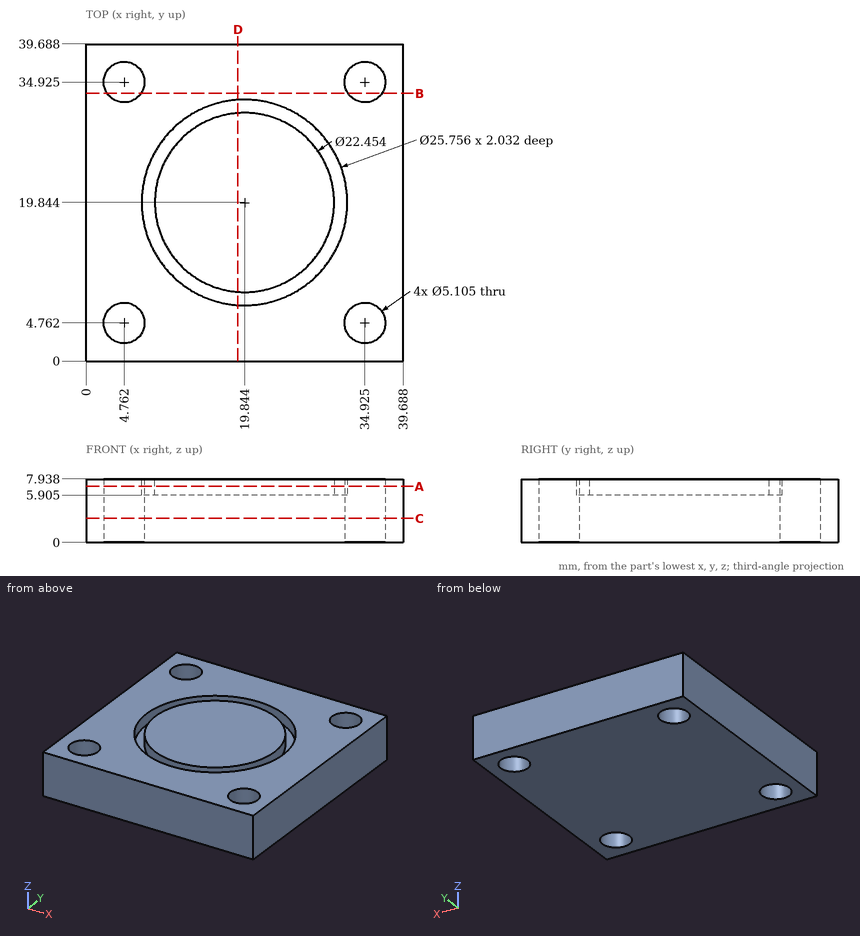
Geometry: see drawing. Coordinates: mm, zero at the bounding-box minimum. Coordinates: 2 decimals unless noted, no trailing zeros. Write each loop counter-clockwise with the first axis right and the second up, starting at its lowest first coordinate (ties: lowest second). Pieces come first, ordered by that corner, then holes. Notation, with made-up numbers: M 70,33 L 82,33 A26 ccw 82,67 Z; hole C 6.25,16.25 d7. An arc over 180 degrees is marked long. Use CSV: the item, a comma, the result in double quotes. Start each with the question number.
1. Ray query, probe 1 along X at (y, z) = (28, 7) (1 decimal); probe 2 along Y at (x, z) = (3.5, 5.5) (1 decimal); probe 3 along X at (y, z) = (34.5, 4) (1 decimal). Return the intervals inside material, ascending.
2. Cut plane C-C on z = 3. Return the cut outline in (x, y) (1 decimal), plus the area to 3 significant figures.
3. Cut plane A-A on z = 7. Return the cut outline in (x, y) (1 decimal).
4. Cut plane B-B on y = 33.5. Return the cut outline in (x, z) (1 decimal).
5. Cut plane D-D on x = 19. Return the cut outline in (y, z) (1 decimal).
Entries:
1,probe 1,"0 to 9.9, 12.1 to 27.6, 29.8 to 39.7"
1,probe 2,"0 to 2.5, 7 to 32.7, 37.1 to 39.7"
1,probe 3,"0 to 2.2, 7.3 to 32.4, 37.4 to 39.7"
2,outline,"M 0,0 L 39.7,0 L 39.7,39.7 L 0,39.7 Z; hole C 4.8,4.8 d5.1; hole C 4.8,34.9 d5.1; hole C 34.9,4.8 d5.1; hole C 34.9,34.9 d5.1"
2,area,"1,490 mm²"
3,outline,"M 0,0 L 39.7,0 L 39.7,39.7 L 0,39.7 Z; C 19.8,19.8 d22.5; hole C 4.8,4.8 d5.1; hole C 4.8,34.9 d5.1; hole C 19.8,19.8 d25.8; hole C 34.9,4.8 d5.1; hole C 34.9,34.9 d5.1"
4,outline,"M 0,0 L 2.6,0 L 2.6,7.9 L 0,7.9 Z; M 6.9,0 L 32.8,0 L 32.8,7.9 L 6.9,7.9 Z; M 37,0 L 39.7,0 L 39.7,7.9 L 37,7.9 Z"
5,outline,"M 0,0 L 39.7,0 L 39.7,7.9 L 32.7,7.9 L 32.7,5.9 L 31,5.9 L 31,7.9 L 8.6,7.9 L 8.6,5.9 L 7,5.9 L 7,7.9 L 0,7.9 Z"
